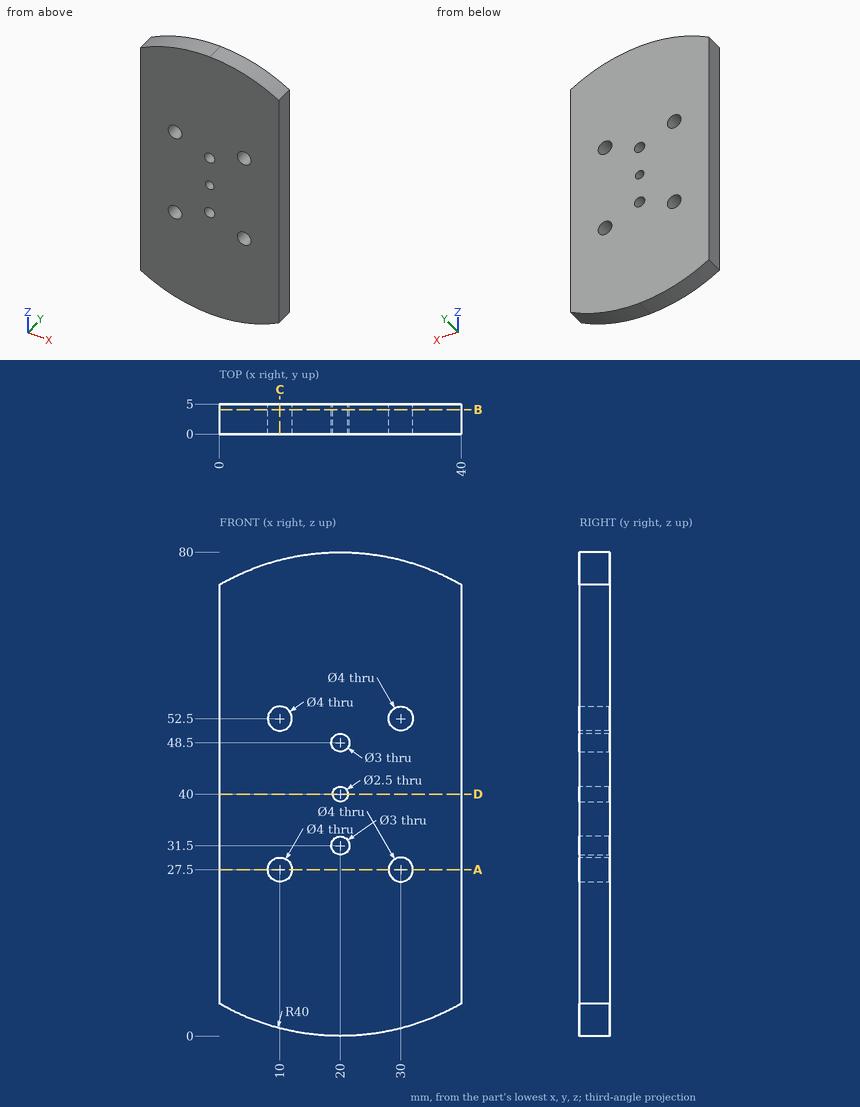
Could you check a few things on this drawing? It's one solid part, dimensions in mm from its lowest x, y, z. Coordinates: 2 decimals unless noted, no trailing zeros. Order: outer loops, then holes, each group sorted by start corner. A loop starts at its lowest first (then second) coordinate and runs counter-clockwise, first axis right, second up. Notation, with made-up numbers: M 14.5,17 L 21.5,17 A16 cw 21.5,32 Z; hole C 43,46.25 d7. An arc over 180 degrees is marked long. Answer as a JSON object with one key per item and string values. Group by question number.
(1) For pin 1 (1 mm diameter, centred on x = 14, y = 1, fed in from +Z); pin 2 (1 mm diameter, centred on x = 28.5, y = 4, fed in from -Z), each with a flat end and sliding along its axis, tell me the tip position at first contact or that it passes through.
(2) Suppose I cut it at B-B, the plane y = 4.05. Please give me the cut outline in (x, z).
(3) Suppose I cut it at C-C, the plane x = 10. Please give me the cut outline in (y, z).
(4) Suppose I cut it at D-D, the plane z = 40. Please give me the cut outline in (x, y), then the cut area to 4 significant figures.
(5) I need wall thicknesses on probe 1 along X at (y, z) = (3.95, 52.5); probe 2 along X at (y, z) = (1.75, 40); probe 3 along Z at (x, y) = (28.5, 0.65). Which ranges of each line are inside material? Lowest first, please.
(6) Suppose I cut it at A-A, the plane z = 27.5. Please give me the cut outline in (x, y), then the cut area to 3 significant figures.
Values found:
{
 "1": {"pin 1": "stops at z = 79.62", "pin 2": "stops at z = 0.81"},
 "2": {"outline": "M 0,5.36 A40 ccw 40,5.36 L 40,74.64 A40 ccw 0,74.64 Z; hole C 10,27.5 d4; hole C 10,52.5 d4; hole C 20,31.5 d3; hole C 20,48.5 d3; hole C 20,40 d2.5; hole C 30,27.5 d4; hole C 30,52.5 d4"},
 "3": {"outline": "M 0,1.27 L 5,1.27 L 5,25.5 L 0,25.5 Z; M 0,29.5 L 5,29.5 L 5,50.5 L 0,50.5 Z; M 0,54.5 L 5,54.5 L 5,78.73 L 0,78.73 Z"},
 "4": {"outline": "M 0,0 L 18.75,0 L 18.75,5 L 0,5 Z; M 21.25,0 L 40,0 L 40,5 L 21.25,5 Z", "area": "187.5 mm^2"},
 "5": {"probe 1": "x = 0 to 8, 12 to 28, 32 to 40", "probe 2": "x = 0 to 18.75, 21.25 to 40", "probe 3": "z = 0.91 to 26.18, 28.82 to 51.18, 53.82 to 79.09"},
 "6": {"outline": "M 0,0 L 8,0 L 8,5 L 0,5 Z; M 12,0 L 28,0 L 28,5 L 12,5 Z; M 32,0 L 40,0 L 40,5 L 32,5 Z", "area": "160 mm^2"}
}
